Build history of the part. All positions in model axes, mm. Face numbers are marked on the shaded views. A direction names the side the tool comes from. Coordinates: 2 decimals unless noted, no trailing zeros. Order: outer loops, then holes, each group sorted by start corner. A loop starts at its lowest first (then second) coordinate and runs counter-clockwise, first axis right, second up. Notation, with made-up numbers: (-7, 57.25) - (45, 57.25) arc R28 cw to (45, 83.25) - close; hole circle Ø4 at (36, -11.5). An arc over 180 degrees is marked (long way). Write each question's results on one line, items separated by ' | '. Start each with the question number.
from build123d import *

# Parameters (mm, degrees)
SKETCH1_W                       = 24.3
SKETCH1_H                       = 24.3
SKETCH1_W_2                     = 14.3
SKETCH1_H_2                     = 14.3
BOSS_EXTRUDE1_DEPTH             = 4
SKETCH3_R                       = 1.5
BOSS_EXTRUDE4_DEPTH             = 4
BOSS_EXTRUDE5_DEPTH             = 4
BOSS_EXTRUDE6_REACH             = 23.355
BOSS_EXTRUDE6_DIRECTION_2_REACH = 23.355
CUT_EXTRUDE1_DEPTH              = 11
SKETCH7_W                       = 24.3
SKETCH7_H                       = 23.3
SKETCH7_W_2                     = 14.3
SKETCH7_H_2                     = 14.3
BOSS_EXTRUDE8_DEPTH             = 1


with BuildPart() as part:
    # Sketch1 → Boss-Extrude1 (new body)
    with BuildSketch(Plane.XY):
        Rectangle(SKETCH1_W, SKETCH1_H)
        Rectangle(SKETCH1_W_2, SKETCH1_H_2, mode=Mode.SUBTRACT)
    extrude(amount=BOSS_EXTRUDE1_DEPTH)

    # Sketch3 → Boss-Extrude4 (add)
    with BuildSketch(Plane(origin=(0, 0, 0), x_dir=(-1, 0, 0), z_dir=(0, 0, -1))):
        with Locations(Location((8.75, 0, 0), (0, 0, 180))):
            Circle(SKETCH3_R)
        with Locations(Location((-8.75, 0, 0), (0, 0, 180))):
            Circle(SKETCH3_R)
    extrude(amount=BOSS_EXTRUDE4_DEPTH)

    # Sketch4 → Boss-Extrude5 (add)
    with BuildSketch(Plane.XY.offset(4)):
        with BuildLine():
            Line((11.248190336, -0.201777492), (11.248190336, -11.15))
            Line((11.248190336, -11.15), (14.15, -11.15))
            Line((14.15, -11.15), (14.15, 13.85))
            Line((14.15, 13.85), (-14.15, 13.85))
            Line((-14.15, 13.85), (-14.15, -11.15))
            Line((-14.15, -11.15), (-11.248190336, -11.15))
            Line((-11.248190336, -11.15), (-11.248190336, -0.201777492))
            ThreePointArc((-11.248190336, -0.201777492), (0, 11.25), (11.248190336, -0.201777492))
        make_face()
    extrude(amount=BOSS_EXTRUDE5_DEPTH)

    # Boss-Extrude6: up to this face of the body (flat: up to its plane)
    boss_extrude6_end = Plane(part.part.faces().sort_by_distance((0, 12.15, 2))[0])
    # Sketch5 → Boss-Extrude6 (add, up to the picked face)
    with BuildSketch(Plane(origin=(0, 0, 0), x_dir=(1, 0, 0), z_dir=(0, 1, 0)), mode=Mode.PRIVATE) as boss_extrude6_sk1:
        Polygon((-12.15, 0), (-14.15, -4), (-12.15, -4), align=None)
    boss_extrude6_tool1 = split(extrude(boss_extrude6_sk1.sketch, amount=BOSS_EXTRUDE6_REACH, mode=Mode.PRIVATE), bisect_by=boss_extrude6_end, keep=Keep.BOTH, mode=Mode.PRIVATE)
    # Sketch5 → Boss-Extrude6 (add, up to the picked face)
    with BuildSketch(Plane(origin=(0, 0, 0), x_dir=(1, 0, 0), z_dir=(0, 1, 0)), mode=Mode.PRIVATE) as boss_extrude6_sk2:
        Polygon((12.15, 0), (12.15, -4), (14.15, -4), align=None)
    boss_extrude6_tool2 = split(extrude(boss_extrude6_sk2.sketch, amount=BOSS_EXTRUDE6_REACH, mode=Mode.PRIVATE), bisect_by=boss_extrude6_end, keep=Keep.BOTH, mode=Mode.PRIVATE)
    add(boss_extrude6_tool1.solids().sort_by(Axis((-12.816667, 0, 2.666667), (0, 1, 0)))[0])
    add(boss_extrude6_tool2.solids().sort_by(Axis((12.816667, 0, 2.666667), (0, 1, 0)))[0])

    # Boss-Extrude6 direction 2: up to this face of the body (flat: up to its plane)
    boss_extrude6_direction_2_end = Plane(part.part.faces().sort_by_distance((12.699095168, -11.15, 6))[0])
    # Sketch5 → Boss-Extrude6 direction 2 (add, up to the picked face)
    with BuildSketch(Plane(origin=(0, 0, 0), x_dir=(1, 0, 0), z_dir=(0, 1, 0)), mode=Mode.PRIVATE) as boss_extrude6_direction_2_sk1:
        Polygon((-12.15, 0), (-14.15, -4), (-12.15, -4), align=None)
    boss_extrude6_direction_2_tool1 = split(extrude(boss_extrude6_direction_2_sk1.sketch, amount=-BOSS_EXTRUDE6_DIRECTION_2_REACH, mode=Mode.PRIVATE), bisect_by=boss_extrude6_direction_2_end, keep=Keep.BOTH, mode=Mode.PRIVATE)
    # Sketch5 → Boss-Extrude6 direction 2 (add, up to the picked face)
    with BuildSketch(Plane(origin=(0, 0, 0), x_dir=(1, 0, 0), z_dir=(0, 1, 0)), mode=Mode.PRIVATE) as boss_extrude6_direction_2_sk2:
        Polygon((12.15, 0), (12.15, -4), (14.15, -4), align=None)
    boss_extrude6_direction_2_tool2 = split(extrude(boss_extrude6_direction_2_sk2.sketch, amount=-BOSS_EXTRUDE6_DIRECTION_2_REACH, mode=Mode.PRIVATE), bisect_by=boss_extrude6_direction_2_end, keep=Keep.BOTH, mode=Mode.PRIVATE)
    add(boss_extrude6_direction_2_tool1.solids().sort_by(Axis((-12.816667, 0, 2.666667), (0, -1, 0)))[0])
    add(boss_extrude6_direction_2_tool2.solids().sort_by(Axis((12.816667, 0, 2.666667), (0, -1, 0)))[0])

    # Sketch6 → Cut-Extrude1 (cut)
    with BuildSketch(Plane.XY.offset(4)):
        Polygon((-14.15, -11.15), (-17.465023318, -11.15), (-17.465023318, -14.474968539), (16.848397365, -14.474968539), (16.848397365, -10.738940706), (14.15, -11.15), align=None)
    extrude(amount=-CUT_EXTRUDE1_DEPTH, mode=Mode.SUBTRACT)

    # Sketch7 → Boss-Extrude8 (add)
    with BuildSketch(Plane(origin=(0, 0, 0), x_dir=(-1, 0, 0), z_dir=(0, 0, -1))):
        with Locations((0, 0.5)):
            Rectangle(SKETCH7_W, SKETCH7_H)
        Rectangle(SKETCH7_W_2, SKETCH7_H_2, mode=Mode.SUBTRACT)
    extrude(amount=BOSS_EXTRUDE8_DEPTH)


solid = part.part
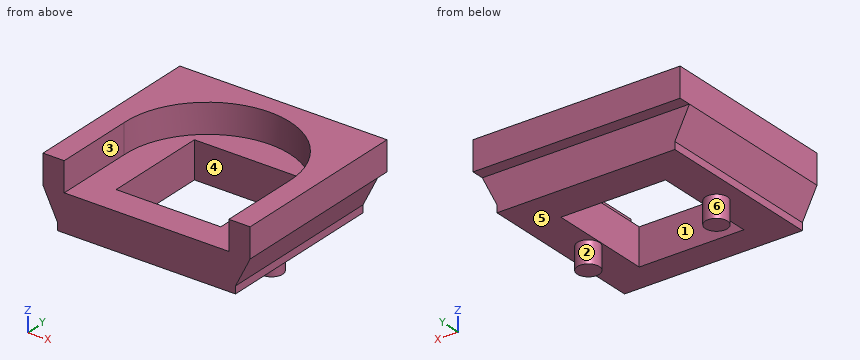
Item 1: Flat gauge pins, fed straight in: P1, Ø1.1, axis at y = -1, z = -0.5, coming from the -X side (3 decimals); P2, Ø11.5, axis at x = 3.5, y = 2.5, coming from the -Z side; P3, Ø5, axis at y = -8.5, z = -2, coming from the +X side; P4, Ø4, axis at x = -6, y = -4.5, coming from the +Z side. Where does each tip first touch, or does it go through?
Item 2: Which spindle directions (+Z, -Z, +X, -X, +Y, -Y) get a long thin tool onto all of the face, cutting with end or side? Do the marked faces 1, 2 and 3. Say none if no direction does.
Item 3: Pull direction Y, two halves, no side cores. Call the marked faces 4, 5 and 6: released by +Y, released by -Y, zero draft, split by the parting line, or undercut.
Item 4: Slice it at B-B (z = -2.75). Write the cut outline in (x, y).
Item 5: Probe probe 1 along Y at (x, z) = (6.75, 1); probe 2 along X at (y, z) = (-1.5, -0.25); probe 3 along Z at (x, y) = (-5.25, 10.5). List the from-to ranges inside material, lowest first.
Item 6: Slice it at A-A (x = 0). Write the cut outline in (y, z).
Item 7: Slice it at D-D (x = -9.75). Write the cut outline in (y, z).
Resolved:
1) P1: x = -12.175 | P2: z = -4 | P3: x = 12.4 | P4: z = 4
2) face 1: +Z, -Z | face 2: -Z | face 3: +Z, -Y
3) face 4: undercut | face 5: zero draft | face 6: split by the parting line
4) outline: circle Ø3 at (-8.75, 0); circle Ø3 at (8.75, 0)
5) probe 1: -11.15 to -7.15, 7.15 to 12.15 | probe 2: -12.15 to -7.15, 7.15 to 12.15 | probe 3: -1 to 8
6) outline: (-11.15, -1) - (-7.15, -1) - (-7.15, 4) - (-11.15, 4) - close; (7.15, -1) - (12.15, -1) - (12.15, 4) - (13.85, 4) - (13.85, 8) - (11.25, 8) - (11.25, 4) - (7.15, 4) - close
7) outline: (-11.15, -1) - (-1.12, -1) - (-1.12, -4) - (1.12, -4) - (1.12, -1) - (12.15, -1) - (12.15, 4) - (13.85, 4) - (13.85, 8) - (5.61, 8) - (5.61, 4) - (-11.15, 4) - close
